Autodesk Inventor part; units mm, degrees
ref_plane "YZ Plane" through (0, 0, 0) normal (1, 0, 0) x (0, 1, 0)
ref_plane "XZ Plane" through (0, 0, 0) normal (0, 1, 0) x (-1, 0, 0)
ref_plane "XY Plane" through (0, 0, 0) normal (0, 0, 1) x (1, 0, 0)
sketch "Sketch1" plane through (0, 0, 0) normal (0, 1, 0) x (-1, 0, 0)
  line L0 (0, 0) -> (4.95, 0)
  line L1 (0, 0) -> (0, -4.95)
  line L2 (0, -4.95) -> (4.95, 0)
  dimension "d0" = 4.95
  dimension "d1" = 4.95
extrude "Extrusion1" add sketch "Sketch1" along normal blind 6
sketch "Sketch2" plane through (0, 6, 0) normal (0, 1, 0) x (1, 0, 0)
  line L0 (-4.95, 0) -> (0, 0)
  line L1 (0, 0) -> (-10, 0)
  line L2 (0, 0) -> (0, 10)
  line L3 (0, 10) -> (-10, 0)
  dimension "d4" = 10
  dimension "d5" = 10
extrude "Extrusion2" add sketch "Sketch2" along normal blind 2
sketch "Sketch3" plane through (0, 8, 0) normal (0, 1, 0) x (1, 0, 0)
  line L0 (-10, 0) -> (-4.95, 0)
  line L1 (-10, 0) -> (-4.95, 0)
  line L2 (0, 4.95) -> (0, 10)
  line L3 (-4.95, 0) -> (0, 4.95)
  line L4 (0, 4.95) -> (0, 10)
  line L5 (0, 10) -> (-10, 0)
  point P0 (0, 0)
extrude "Extrusion3" add sketch "Sketch3" along normal blind 19.75
sketch "Sketch4" plane through (0, 27.75, 0) normal (0, 1, 0) x (1, 0, 0)
  line L0 (-4.95, 0) -> (0, 0)
  line L1 (-4.95, 0) -> (0, 0)
  line L2 (-4.95, 0) -> (0, 4.95)
  line L3 (0, 0) -> (0, 4.95)
extrude "Extrusion4" add sketch "Sketch4" against normal blind 5
sketch "Sketch6" plane through (0, 27.75, 0) normal (0, 1, 0) x (1, 0, 0)
  line L0 (-10, 0) -> (-4.95, 0)
  line L1 (-10, 0) -> (0, 10)
  line L2 (0, 10) -> (-10, 0)
  line L3 (-4.95, 0) -> (0, 0)
  line L4 (0, 0) -> (0, 10)
  circle A0 centre (-2.6665, 2.6666) radius 1.25
  dimension "d12" = 2.5
  dimension "d17" = 3.3
  dimension "d18" = 2.6665
  dimension "d19" = 2.6666
extrude "Extrusion5" cut sketch "Sketch6" against normal blind 5 contours A0
sketch "Sketch7" plane through (0, 8, 0) normal (0, 1, 0) x (1, 0, 0)
  line L0 (0, 4.95) -> (-4.95, 0)
  line L1 (0, 4.95) -> (-4.95, 0)
  line L2 (0, 4.95) -> (-4.95, 0)
  line L3 (0, 0) -> (0, 4.95)
  line L4 (-4.95, 0) -> (0, 0)
  line L5 (0, 0) -> (0, 4.95)
extrude "Extrusion6" add sketch "Sketch7" along normal blind 2
sketch "Sketch8" plane through (0, 0, 0) normal (0, -1, 0) x (1, 0, 0)
  line L0 (-4.95, 0) -> (0, 0)
  line L1 (0, 0) -> (0, -4.95)
  circle A0 centre (-1.45, -1.45) radius 1
  dimension "d20" = 1.45
  dimension "d21" = 1.45
  dimension "d22" = 2
extrude "Extrusion7" cut sketch "Sketch8" against normal up to surface (10 mm away)
sketch "Sketch9" plane through (0, 27.75, 0) normal (0, 1, 0) x (1, 0, 0)
  line L0 (0, 10) -> (10.5977, -0.5977)
  line L1 (0, 0) -> (0, 10)
  line L2 (0, 10) -> (-10, 0)
  line L3 (0, 10) -> (11.6673, -1.6673)
  line L4 (11.6673, -1.6673) -> (1.6673, -11.6673)
  line L5 (11.6673, -1.6673) -> (30.5491, -1.6673) construction
  line L6 (-10, 0) -> (1.6673, -11.6673)
  arc A0 (8.435, -4.8995) -> (4.8995, -8.435) centre (6.6673, -6.6673) ccw
  line L7 (6.6673, -6.6673) -> (4.8995, -4.8995)
  circle A1 centre (4.8995, -4.8995) radius 1.25
  point P0 (10.5977, -0.5977)
  dimension "d25" = 45
  dimension "d26" = 16.5
  dimension "d27" = 135
  dimension "d28" = 5
  dimension "d29" = 2.5
extrude "Extrusion8" add sketch "Sketch9" against normal up to surface (5 mm away) contours L0 L3 L4 A0 A1 L6 L2 | L4 L7 A1 A0 | A0 A1 L7 L4
sketch "Sketch10" plane through (0, 6, 0) normal (0, -1, 0) x (1, 0, 0)
  line L0 (0, -4.95) -> (-4.95, 0)
  line L1 (-10, 0) -> (-4.95, 0)
  line L2 (0, -10) -> (-10, 0)
  line L3 (0, -4.95) -> (0, -10)
  point P0 (0, 0)
extrude "Extrusion9" add sketch "Sketch10" along normal blind 3
sketch "Sketch11" plane through (0, 10, 0) normal (0, 1, 0) x (1, 0, 0)
  line L0 (0, 0) -> (0, 4.95)
  line L1 (-4.95, 0) -> (0, 4.95)
  line L2 (-4.95, 0) -> (0, 0)
extrude "Extrusion10" cut sketch "Sketch11" against normal blind 4
properties part number "bracket servo left_3DPrint"
Could you check a few things on this model? Use its own coordinates, in mm. A direction names the side the tool comes from. Give positions to 0.01 mm unless a question says otherwise; leave off trailing zeros. Order: outer loops, then holes, each group sorted by start corner. A loop starts at its lowest first (then second) coordinate and runs counter-clockwise, first axis right, second up.
Item 1: I need wall thicknesses on line 1 (Y direction, x = 3, z = -3.5); line 2 (Z direction, x = -1.45, y = 1.8); line 3 (Z direction, x = -0.25, y = 7.5). Which ranges of each line are inside material? Lowest first, please.
Item 2: I'm going to push flat-ended pins straight in: pin 1 (5 mm diameter, centred on y = 7, z = -5, fed in from +X); pin 2 (2 mm diameter, centred on x = -1.5, y = 16.5, fed in from +Z); pin 3 (5 mm diameter, centred on x = 2, z = -8, fed in from -Y); pin 4 (1 mm diameter, centred on x = 1.5, y = 20, fed in from +Z). Where does each tip first touch, or does it pass through?
Item 3: For faces 4 (the face through (-6, 11, 0)), 5 (the face through (-4, 3, -4)), 6 (the face through (-2.187, 2.958, -0.774)), 7 (the face through (-2.51, 14.49, -2.44)), 8 (the face through (0, 12, -6)), which set-ups out of +Z, -Z, +X, -X, +Y, -Y let a thin tool reach every point of the face, with its end or its side?
Item 4: If we section it at A-A, the plane x = -1.45: Write out the boundary of the cut face in (y, z), plus the area to 3 significant figures.
Item 5: If we section it at B-B, the plane z = -1.45: Write out the boundary of the cut face in (x, y), plus the area to 3 significant figures.
Item 6: If we section it at C-C, the plane y = 8: Write out the boundary of the cut face in (x, z).
Item 7: If we section it at D-D, the plane x = -7.5: Write out the boundary of the cut face in (y, z), plus the area to 3 significant figures.
Item 8: If we mould it in two halves opening along Z, with no side actions, what happens to faces 1 (the face through (-2.1, 6, -2.5)), 2 (the face through (-5, 16, -5)), 3 (the face through (3.65, 25.28, 4.84))? For each: pulls with the +Z half, pulls with the -Z half, needs draft (parallel to the pull), parting line crosses it, or undercut.
Values:
1. line 1: y = 22.75 to 27.75
1. line 2: z = -3.5 to -2.45, -0.45 to 0
1. line 3: z = -9.75 to -4.7
2. pin 1: stops at x = 0
2. pin 2: stops at z = -2.45
2. pin 3: stops at y = 3
2. pin 4: passes through
3. face 4: +Z, +X, -X, -Y
3. face 5: -Z, -X, -Y
3. face 6: -Y
3. face 7: +Z, +X
3. face 8: +Z, -Z, +X, -Y
4. outline: (0, -3.5) - (3, -3.5) - (3, -8.55) - (27.75, -8.55) - (27.75, 8.55) - (22.75, 8.55) - (22.75, -3.5) - (6, -3.5) - (6, -2.45) - (0, -2.45) - close; (0, -0.45) - (6, -0.45) - (6, 0) - (0, 0) - close
4. area: 194 mm2
5. outline: (-8.55, 3) - (-3.5, 3) - (-3.5, 0) - (-2.45, 0) - (-2.45, 6) - (-3.5, 6) - (-3.5, 22.75) - (8.55, 22.75) - (8.55, 27.75) - (-8.55, 27.75) - close; (-0.45, 0) - (0, 0) - (0, 6) - (-0.45, 6) - close
5. area: 194 mm2
6. outline: (-10, 0) - (0, -10) - (0, -4.95) - (-4.95, 0) - close
7. outline: (3, -2.5) - (27.75, -2.5) - (27.75, 2.5) - (22.75, 2.5) - (22.75, 0) - (3, 0) - close
7. area: 74.4 mm2
8. face 1: needs draft
8. face 2: pulls with the -Z half
8. face 3: undercut
